```python
from build123d import *

# Parameters (mm, degrees)
SKETCH1_R           = 1.5
BOSS_EXTRUDE1_DEPTH = 3


with BuildPart() as part:
    # Sketch1 → Boss-Extrude1 (new body)
    with BuildSketch(Plane(origin=(0, 0, 0), x_dir=(1, 0, 0), z_dir=(0, 1, 0))):
        with BuildLine():
            Line((234.205080757, -100), (234.205080757, 100))
            ThreePointArc((234.205080757, 100), (203.705080757, 152.827549631), (142.705080757, 152.827549631))
            Line((142.705080757, 152.827549631), (-30.5, 52.827549631))
            ThreePointArc((-30.5, 52.827549631), (-61, 0), (-30.5, -52.827549631))
            Line((-30.5, -52.827549631), (142.705080757, -152.827549631))
            ThreePointArc((142.705080757, -152.827549631), (203.705080757, -152.827549631), (234.205080757, -100))
        make_face()
        with Locations((53.582540378, -59.525)):
            Circle(SKETCH1_R, mode=Mode.SUBTRACT)
        with Locations((80.524854378, -15.531728)):
            Circle(SKETCH1_R, mode=Mode.SUBTRACT)
        with Locations((116.913429378, -67.500001)):
            Circle(SKETCH1_R, mode=Mode.SUBTRACT)
        with Locations((53.582540378, 40.475)):
            Circle(SKETCH1_R, mode=Mode.SUBTRACT)
        with Locations((80.524854378, 84.468272)):
            Circle(SKETCH1_R, mode=Mode.SUBTRACT)
        with Locations((116.913429378, 32.499999)):
            Circle(SKETCH1_R, mode=Mode.SUBTRACT)
        with Locations((203.515969757, -17.500001)):
            Circle(SKETCH1_R, mode=Mode.SUBTRACT)
        with Locations((140.185080757, -9.525)):
            Circle(SKETCH1_R, mode=Mode.SUBTRACT)
        with Locations((167.127394757, 34.468272)):
            Circle(SKETCH1_R, mode=Mode.SUBTRACT)
        with Locations((-6.077686, 34.468272)):
            Circle(SKETCH1_R, mode=Mode.SUBTRACT)
        with Locations((-33.02, -9.525)):
            Circle(SKETCH1_R, mode=Mode.SUBTRACT)
        with Locations((30.310889, -17.500001)):
            Circle(SKETCH1_R, mode=Mode.SUBTRACT)
        with Locations((167.127394757, 134.468272)):
            Circle(SKETCH1_R, mode=Mode.SUBTRACT)
        with Locations((140.185080757, 90.475)):
            Circle(SKETCH1_R, mode=Mode.SUBTRACT)
        with Locations((203.515969757, 82.499999)):
            Circle(SKETCH1_R, mode=Mode.SUBTRACT)
        with Locations((167.127394757, -65.531728)):
            Circle(SKETCH1_R, mode=Mode.SUBTRACT)
        with Locations((140.185080757, -109.525)):
            Circle(SKETCH1_R, mode=Mode.SUBTRACT)
        with Locations((203.515969757, -117.500001)):
            Circle(SKETCH1_R, mode=Mode.SUBTRACT)
    extrude(amount=BOSS_EXTRUDE1_DEPTH)


solid = part.part
```
Here's how the part is built. I have some questions about the finished solid (model axes, mm). Round coordinates to 2 decimals unless told otherwise and drop trailing zeros. Order: outer loops, then holes, each group sorted by start corner. A loop starts at its lowest first (then second) coordinate and runs counter-clockwise, first axis right, second up. Notation, with made-up numbers: (-29, 58) -> (21, 58) arc R24 cw to (21, 84) -> close; hole circle Ø11 at (-3.5, 19). An arc over 180 degrees is marked (long way). Use a Markdown table: item, result. Add a question column.
(1) I need wall thicknesses on line 1 along Z through (x, y) = (-48, 1.85); line 2 along X through (y, z) = (2.05, -68); line 3 along X through (y, z) = (2.5, -46.5). Which ranges of each line are inside material? Lowest first, please.
(2) Suppose I cut it at A-A, the plane y = 1.4. Count the separate pieces of the cut face and the enclosed holes in it, and give its area (3 significant figures).
(3) Suppose I cut it at B-B, the plane z = -27. Please give me the cut outline in (x, y), and give its area (3 significant figures).
(4) If we mould it in two halves opening along X, with no side actions, what happens to faces 1 (the face through (117, 0, -2)), 2 (the face through (202.927, 1.479, 153.269)), 3 (the face through (-60.993, 1.479, -0.894))? For each: released by +X, released by -X, zero draft, split by the parting line, or undercut.
(5) Suppose I cut it at C-C, the plane x = 39. Please give me the cut outline in (y, z).
(6) For pin 1 Ø2.5 at (x, z) = (53.58, 59.52) entering from +Y, with a flat end and sliding along its axis, tell me the tip position at first contact or that it passes through.
Verdict:
| question | item | result |
|---|---|---|
| 1 | line 1 | -37.64 to 37.64 |
| 1 | line 2 | -4.22 to 234.21 |
| 1 | line 3 | -39.48 to 234.21 |
| 2 | separate pieces | 1 |
| 2 | enclosed holes | 18 |
| 2 | area | 65,500 mm2 |
| 3 | outline | (-54.7, 0) -> (234.21, 0) -> (234.21, 3) -> (-54.7, 3) -> close |
| 3 | area | 867 mm2 |
| 4 | face 1 | zero draft |
| 4 | face 2 | split by the parting line |
| 4 | face 3 | released by -X |
| 5 | outline | (0, -92.95) -> (3, -92.95) -> (3, 92.95) -> (0, 92.95) -> close |
| 6 | pin 1 | through |
